Here's how the part is built. I have some questions about the finished solid (model axes, mm). A direction names the side the tool comes from. Coordinates: 2 decimals unless noted, no trailing zeros. Write each loop counter-clockwise with the first axis right and the second up, starting at its lowest first coordinate (ties: lowest second). Pieces come first, ordered by that corner, then holes. Notation, with made-up numbers: (31, 5.25) -> (57, 5.25) arc R15 cw to (57, 23.25) -> close; hole circle Ø2 at (-32.75, 85). An arc over 180 degrees is marked (long way). Use a Markdown table: item, result. Add a question column.
```python
from build123d import *

# Parameters (mm, degrees)
SKETCH1_W           = 7.5
SKETCH1_H           = 18
BOSS_EXTRUDE1_DEPTH = 0.7
SKETCH2_R           = 1
BOSS_EXTRUDE2_DEPTH = 18
SKETCH4_R           = 0.75
CUT_EXTRUDE1_DEPTH  = 20.602295784
CUT_EXTRUDE2_START  = -4.5
SKETCH5_R           = 1
CUT_EXTRUDE2_DEPTH  = 4.5
LPATTERN1_COUNT     = 2
LPATTERN1_PITCH     = 9
SKETCH6_R           = 1.5
CUT_EXTRUDE3_DEPTH  = 20.543285292


with BuildPart() as part:
    # Sketch1 → Boss-Extrude1 (new body)
    with BuildSketch(Plane(origin=(0, 0, 0), x_dir=(1, 0, 0), z_dir=(0, 1, 0))):
        with Locations((3.75, 9)):
            Rectangle(SKETCH1_W, SKETCH1_H)
    extrude(amount=BOSS_EXTRUDE1_DEPTH)

    # Sketch2 → Boss-Extrude2 (add, through all)
    with BuildSketch(Plane.XY):
        with Locations((0, 1)):
            Circle(SKETCH2_R)
    extrude(amount=-BOSS_EXTRUDE2_DEPTH)

    # Sketch4 → Cut-Extrude1 (cut, through all)
    with BuildSketch(Plane.XY):
        with Locations((0, 1)):
            Circle(SKETCH4_R)
    extrude(amount=-CUT_EXTRUDE1_DEPTH, mode=Mode.SUBTRACT)

    # Sketch5 → Cut-Extrude2 (cut)
    with BuildSketch(Plane.XY.offset(CUT_EXTRUDE2_START)):
        with Locations((0, 1)):
            Circle(SKETCH5_R)
    cut_extrude2 = extrude(amount=-CUT_EXTRUDE2_DEPTH, mode=Mode.SUBTRACT)

    # LPattern1: Cut-Extrude2 ×2
    with Locations(*[(0, 0, -i * LPATTERN1_PITCH) for i in range(1, LPATTERN1_COUNT)]):
        add(cut_extrude2, mode=Mode.SUBTRACT)

    # Sketch6 → Cut-Extrude3 (cut, through all)
    with BuildSketch(Plane(origin=(0, 0.7, 0), x_dir=(1, 0, 0), z_dir=(0, 1, 0))):
        with Locations(Location((5, 2.5, 0), (0, 0, 270))):
            Circle(SKETCH6_R)
        with Locations(Location((5, 15.5, 0), (0, 0, 90))):
            Circle(SKETCH6_R)
    extrude(amount=-CUT_EXTRUDE3_DEPTH, mode=Mode.SUBTRACT)


solid = part.part
```
Q1. Suppose I cut it at C-C, the plane x = 5.5. Write out the boundary of the cut face in (y, z).
Q2. Will these pins go through, and if not, where does the flat tip stop? pin 1 (1 mm diameter, centred on x = 4, y = 1.5, fed in from +Z); pin 2 (1 mm diameter, centred on x = 0.5, y = 1.5, fed in from -Z); pin 3 (5 mm diameter, centred on x = 3, z = -8.5, fed in from +Y).
Q3. Which directions (+Z, -Z, +X, -X, +Y, -Y) give clear straight access to the entire face, cutting with the end or side of a thin tool? Please do faces 4 (the cylindrical face through (0.6, 0.2, -15.7)), 5 (the flat face through (4, 0, -9)).
Q4. Thinking about a two-plate mould opening in Z: for faces 1 (the cylindrical face through (0.6, 0.2, -6.7)), 2 (the flat face through (3.2, 0.3, 0)), 3 (the cylindrical face through (-0.163, 0.268, -11.218)), which applies, released by +Z, released by -Z, zero draft, split by the parting line, or undercut?
Q5. Suppose I cut it at D-D, the plane z = -15.5. Write out the boundary of the cut face in (x, y).
Q6. Suppose I cut it at B-B, the plane y = 1. Write out the boundary of the cut face in (x, z).
Q7. Suppose I cut it at A-A, the plane z = -1.25. Write out the boundary of the cut face in (x, y), and give its area (3 significant figures).
Q8. Please list where these lines run through material, in increasing order: line 1 (Y direction, x = 0, z = -12.4); line 2 (X direction, y = 0.35, z = -2.5); line 3 (Y direction, x = 1.75, z = -17.25).
Answer key:
| question | item | result |
|---|---|---|
| 1 | outline | (0, -18) -> (0.7, -18) -> (0.7, -16.91) -> (0, -16.91) -> close; (0, -14.09) -> (0.7, -14.09) -> (0.7, -3.91) -> (0, -3.91) -> close; (0, -1.09) -> (0.7, -1.09) -> (0.7, 0) -> (0, 0) -> close |
| 2 | pin 1 | passes through |
| 2 | pin 2 | stops at z = -13.5 |
| 2 | pin 3 | stops at y = 1.83 |
| 3 | face 4 | -Z, -X, +Y |
| 3 | face 5 | +Z, -Z, +X, -X, -Y |
| 4 | face 1 | undercut |
| 4 | face 2 | released by +Z |
| 4 | face 3 | zero draft |
| 5 | outline | (0, 0) -> (3.5, 0) -> (3.5, 0.7) -> (0.95, 0.7) arc R1 cw to start; (6.5, 0) -> (7.5, 0) -> (7.5, 0.7) -> (6.5, 0.7) -> close |
| 6 | outline | (-1, -13.5) -> (-0.75, -13.5) -> (-0.75, -9) -> (-1, -9) -> close; (-1, -4.5) -> (-0.75, -4.5) -> (-0.75, 0) -> (-1, 0) -> close; (0.75, -13.5) -> (1, -13.5) -> (1, -9) -> (0.75, -9) -> close; (0.75, -4.5) -> (1, -4.5) -> (1, 0) -> (0.75, 0) -> close |
| 7 | outline | (0, 0) -> (4.17, 0) -> (4.17, 0.7) -> (0.95, 0.7) arc R1 ccw (long way) to start; (5.83, 0) -> (7.5, 0) -> (7.5, 0.7) -> (5.83, 0.7) -> close; hole circle Ø1.5 at (0, 1) |
| 7 | area | 4.97 mm^2 |
| 8 | line 1 | y = 0 to 0.25, 1.75 to 2 |
| 8 | line 2 | x = -0.76 to -0.37, 0.37 to 3.5, 6.5 to 7.5 |
| 8 | line 3 | y = 0 to 0.7 |
